```python
from build123d import *

# Parameters (mm, degrees)
BASPROSKE_W        = 12
BASPROSKE_H        = 12
TOOTHCUT_DEPTH     = 21.784609691
TEETHCUTS_COUNT    = 10
TEETHCUTS_ANGLE    = 324
BORSKE_R           = 0.4
BORE_DEPTH         = 50.0000508
SCALE1_SCALE       = 0.5
CUT_EXTRUDE1_DEPTH = 11.2470399


with BuildPart() as part:
    # BasProSke → Base-Revolve (revolve)
    with BuildSketch(Plane(origin=(0, 0, 0), x_dir=(1, 0, 0), z_dir=(0, 1, 0)), mode=Mode.PRIVATE) as base_revolve_sk:
        with Locations((6, 6)):
            Rectangle(BASPROSKE_W, BASPROSKE_H)
    revolve(base_revolve_sk.sketch.rotate(Axis((-10, 0, 0), (1, 0, 0)), 180), axis=Axis((-10, 0, 0), (1, 0, 0)))

    # TooCutSke → ToothCut (cut, through all)
    with BuildSketch(Plane(origin=(0, 0, 0), x_dir=(0, 0, -1), z_dir=(1, 0, 0))):
        with BuildLine():
            ThreePointArc((1.173662691, 7.406586048), (0, 7.499), (-1.173662691, 7.406586048))
            ThreePointArc((-1.173662691, 7.406586048), (-1.668191438, 9.834565786), (-3.497907776, 11.50542856))
            ThreePointArc((-3.497907776, 11.50542856), (0, 12.0254), (3.497907776, 11.50542856))
            ThreePointArc((3.497907776, 11.50542856), (1.668191438, 9.834565786), (1.173662691, 7.406586048))
        make_face()
    toothcut = extrude(amount=TOOTHCUT_DEPTH, mode=Mode.SUBTRACT)

    # TeethCuts: ToothCut ×10 about axis
    teethcuts_axis = Axis((-10, 0, 0), (1, 0, 0))
    for i in range(1, TEETHCUTS_COUNT):
        add(toothcut.rotate(teethcuts_axis, i * TEETHCUTS_ANGLE / (TEETHCUTS_COUNT - 1)), mode=Mode.SUBTRACT)

    # BorSke → Bore (cut, symmetric)
    with BuildSketch(Plane(origin=(0, 0, 0), x_dir=(0, 0, -1), z_dir=(1, 0, 0))):
        with Locations(Location((0, 0, 0), (0, 0, 180))):
            Circle(BORSKE_R)
    extrude(amount=BORE_DEPTH, both=True, mode=Mode.SUBTRACT)


with BuildPart() as part_1:
    # Scale1: scaled about (6, 0, 0)
    add(part.part.scale(SCALE1_SCALE).moved(Location((3, 0, 0))))

    # Sketch2 → Cut-Extrude1 (cut, through all)
    with BuildSketch(Plane(origin=(9, 0, 0), x_dir=(0, 0, -1), z_dir=(1, 0, 0))):
        with BuildLine():
            Line((-1.84770017, 1.684043967), (1.09932616, 2.245324474))
            ThreePointArc((1.09932616, 2.245324474), (0.467733756, -2.455855275), (-1.84770017, 1.684043967))
        make_face()
    extrude(amount=-CUT_EXTRUDE1_DEPTH, mode=Mode.SUBTRACT)


solid = part_1.part
```
CAD build for the part. Positions are in the model's coordinates, mm. Round coordinates to 2 decimals unless told otherwise and drop trailing zeros. Loops run counter-clockwise (first coordinate to the right, second up) from the corner with the lowest first, then second, coordinate; pieces in that order, holes last. Notation, with made-up numbers: (12.5, 76) - (18.5, 76) arc R28 cw to (18.5, 106) - close; hole circle Ø2 at (49, -14.5). An arc over 180 degrees is marked (long way). Return JSON: item names as keys, results as strings. Group by question number.
Q1. Drill centre lines: line 1 along Z through (x, y) = (6.85, 0); line 2 along Y through (x, z) = (8, -4.25); line 3 along Z through (x, y) = (6.25, 1). Where is each one in solid material? Low to high. Write a range as [from, to].
Q2. Band-saw the part on B-B on y = -4. Give the cut face in (x, z), plus the area to 3 significant figures.
Q3. Band-saw the part on D-D on z = -4.5. Give the cut face in (x, y), plus the area to 3 significant figures.
Q4. Flat gauge pin, fed straight in: pin 1 Ø1 at (x, z) = (8, 4) entering from +Y. Where does the tip first touch, or does it go through?
Q5. Band-saw the part on C-C on z = 1.25. Give the cut face in (x, y), plus the area to 3 significant figures.
Q6. Band-saw the part on A-A on z = 3.5. Give the cut face in (x, y).
Solutions:
{
 "1": {"line 1": "z = [-6, -2.5], [2.5, 6]", "line 2": "y = [-3.66, -2.15], [-0.75, 0.75], [2.15, 3.66]", "line 3": "z = [-3.61, -2.29], [2.29, 3.61]"},
 "2": {"outline": "(3, -2.1) - (9, -2.1) - (9, -0.58) - (3, -0.58) - close; (3, 0.58) - (9, 0.58) - (9, 2.1) - (3, 2.1) - close", "area": "18.4 mm^2"},
 "3": {"outline": "(3, -3.66) - (9, -3.66) - (9, -2.41) - (3, -2.41) - close; (3, -0.77) - (9, -0.77) - (9, 0.77) - (3, 0.77) - close; (3, 2.41) - (9, 2.41) - (9, 3.66) - (3, 3.66) - close", "area": "24.3 mm^2"},
 "4": {"pin 1": "stops at y = 3.67"},
 "5": {"outline": "(3, -5.43) - (9, -5.43) - (9, -2.17) - (3, -2.17) - close; (3, 1.8) - (9, 1.8) - (9, 5.43) - (3, 5.43) - close", "area": "41.4 mm^2"},
 "6": {"outline": "(3, -3.46) - (9, -3.46) - (9, -1.74) - (3, -1.74) - close; (3, -1.34) - (9, -1.34) - (9, 1.34) - (3, 1.34) - close; (3, 1.74) - (9, 1.74) - (9, 3.46) - (3, 3.46) - close"}
}
